```python
from build123d import *

# Parameters (mm, degrees)
F0_R      = 16.5
F1_DEPTH  = 10
F2_R      = 13
F3_DEPTH  = 10.5
F4_SIZE   = 0.5
F5_R      = 4.95
F6_DEPTH  = 12.5
F7_SIZE   = 0.5
F8_R      = 3.75
F9_DEPTH  = 8
F10_SIZE  = 0.5
F11_R     = 16.5
F11_R_2   = 13
F12_DEPTH = 7
F13_R     = 25
F14_DEPTH = 7
F15_SIZE  = 0.5


with BuildPart() as f1:
    # F0 (on Top) → F1 (new body)
    with BuildSketch(Plane.XY):
        Circle(F0_R)
    extrude(amount=F1_DEPTH)

    # F2 (on face) → F3 (join)
    with BuildSketch(Plane.XY.offset(10)):
        Circle(F2_R)
        with BuildLine():
            ThreePointArc((-7.4852813742, 6.6310302931), (-5, 8.6602540378), (-2, 9.7979589711))
            Line((-2, 9.7979589711), (-2, 8.4))
            Line((-2, 8.4), (2, 8.4))
            Line((2, 8.4), (2, 9.7979589711))
            ThreePointArc((2, 9.7979589711), (5, 8.6602540378), (7.4852813742, 6.6310302931))
            Line((7.4852813742, 6.6310302931), (6.2746133918, 5.9320508076))
            Line((6.2746133918, 5.9320508076), (8.2746133918, 2.4679491924))
            Line((8.2746133918, 2.4679491924), (9.4852813742, 3.166928678))
            ThreePointArc((9.4852813742, 3.166928678), (10, 0), (9.4852813742, -3.166928678))
            Line((9.4852813742, -3.166928678), (8.2746133918, -2.4679491924))
            Line((8.2746133918, -2.4679491924), (6.2746133918, -5.9320508076))
            Line((6.2746133918, -5.9320508076), (7.4852813742, -6.6310302931))
            ThreePointArc((7.4852813742, -6.6310302931), (5, -8.6602540378), (2, -9.7979589711))
            Line((2, -9.7979589711), (2, -8.4))
            Line((2, -8.4), (-2, -8.4))
            Line((-2, -8.4), (-2, -9.7979589711))
            ThreePointArc((-2, -9.7979589711), (-5, -8.6602540378), (-7.4852813742, -6.6310302931))
            Line((-7.4852813742, -6.6310302931), (-6.2746133918, -5.9320508076))
            Line((-6.2746133918, -5.9320508076), (-8.2746133918, -2.4679491924))
            Line((-8.2746133918, -2.4679491924), (-9.4852813742, -3.166928678))
            ThreePointArc((-9.4852813742, -3.166928678), (-10, 0), (-9.4852813742, 3.166928678))
            Line((-9.4852813742, 3.166928678), (-8.2746133918, 2.4679491924))
            Line((-8.2746133918, 2.4679491924), (-6.2746133918, 5.9320508076))
            Line((-6.2746133918, 5.9320508076), (-7.4852813742, 6.6310302931))
        make_face(mode=Mode.SUBTRACT)
    extrude(amount=F3_DEPTH)

    # F4
    f4_edges = [f1.edges().sort_by_distance(p)[0] for p in [
        (0, 8.4, 20.5),
        (-7.274613, 4.2, 20.5),
        (-7.274613, -4.2, 20.5),
        (0, -8.4, 20.5),
        (7.274613, -4.2, 20.5),
        (7.274613, 4.2, 20.5),
    ]]
    chamfer(f4_edges, length=F4_SIZE)

    # F5 (on face) → F6 (join)
    with BuildSketch(Plane.XY.offset(10)):
        Circle(F5_R)
    extrude(amount=F6_DEPTH)

    # F7
    f7_edges = [f1.edges().sort_by_distance(p)[0] for p in [
        (-4.95, 0, 22.5),
    ]]
    chamfer(f7_edges, length=F7_SIZE)

    # F8 (on face) → F9 (join)
    with BuildSketch(Plane.XY.offset(22.5)):
        Circle(F8_R)
    extrude(amount=F9_DEPTH)

    # F10
    f10_edges = [f1.edges().sort_by_distance(p)[0] for p in [
        (-3.75, 0, 30.5),
    ]]
    chamfer(f10_edges, length=F10_SIZE)

    # F11 (on face) → F12 (join)
    with BuildSketch(Plane.XY.offset(10)):
        Circle(F11_R)
        Circle(F11_R_2, mode=Mode.SUBTRACT)
    extrude(amount=F12_DEPTH)

    # F13 (on face) → F14 (cut)
    with BuildSketch(Plane(origin=(0, 0, 0), x_dir=(1, 0, 0), z_dir=(0, 0, -1))):
        Circle(F13_R)
    extrude(amount=-F14_DEPTH, mode=Mode.SUBTRACT)

    # F15
    f15_edges = [f1.edges().sort_by_distance(p)[0] for p in [
        (-13, 0, 20.5),
        (-16.5, 0, 17),
        (-16.5, 0, 7),
    ]]
    chamfer(f15_edges, length=F15_SIZE)


solid = f1.part
```
The listing builds one solid part. Answer for the finished solid, in the listing's coordinates (mm). A direction names the side the tool comes from. Give positions to 0.01 mm unless a question says otherwise; leave off trailing zeros. Loops run counter-clockwise (first coordinate to the right, second up) from the corner with the lowest first, then second, coordinate; pieces in that order, holes last. Notation, with made-up numbers: M 55.25,14.25 L 93.25,14.25 A20 ccw 93.25,48.25 Z; hole C -32.5,50 d2. An arc over 180 degrees is marked long. One line per item, written item: value.
Q1. For faces 1 (the face through (7.289, -4.176, 14.93)), 2 (the face through (0, 0, 7)), determine the directions among +Z, -Z, +X, -X, +Y, -Y from which every point of the face is accessible in a straight line to the end or side of a thin tool.
Working result:
face 1: +Z
face 2: -Z, +X, -X, +Y, -Y
Q2. A cutting plane is placed at B-B on z = 14. Determine the outline of the cut face in (x, y), then the cut area to 3 significant figures.
Working result:
outline: C 0,0 d33; C 0,0 d9.9; hole M -9.49,-3.17 L -8.27,-2.47 L -6.27,-5.93 L -7.49,-6.63 A10 ccw -2,-9.8 L -2,-8.4 L 2,-8.4 L 2,-9.8 A10 ccw 7.49,-6.63 L 6.27,-5.93 L 8.27,-2.47 L 9.49,-3.17 A10 ccw 9.49,3.17 L 8.27,2.47 L 6.27,5.93 L 7.49,6.63 A10 ccw 2,9.8 L 2,8.4 L -2,8.4 L -2,9.8 A10 ccw -7.49,6.63 L -6.27,5.93 L -8.27,2.47 L -9.49,3.17 A10 ccw Z
area: 655 mm^2
Q3. Determine the mould class of faces 3 (the face through (8.888, -2.822, 15.176)), 4 (the face through (0, 0, 30.5)), 5 (the face through (15.24, -6.32, 11.94)) for opening direction Y: +Y half, -Y half, draft (parallel to the pull), parting line (faces both ways), or undercut.
Working result:
face 3: undercut
face 4: draft
face 5: parting line
Q4. Find the intervals of material crossed by line 1 (Y direction, x = -7, z = 14.75); line 2 (Y direction, x = -6.5, z = 16.5); line 3 (Y direction, x = 3, z = 15), in increasing order. Write a range as from..to.
Working result:
line 1: y = -14.94..-7.14, -6.35..-4.68, 4.68..6.35, 7.14..14.94
line 2: y = -15.17..-7.6, -6.06..-5.54, 5.54..6.06, 7.6..15.17
line 3: y = -16.22..-9.54, -3.94..3.94, 9.54..16.22
Q5. Flat-ended cylindrical pins translate along their axes: P1, Ø2, axis at x = -9, y = 11.5, coming from the +Z side; P2, Ø3, axis at x = 0.5, z = 14, coming from the +Y side; P3, Ø5, axis at y = 11, z = 24.5, coming from the -X side; P4, Ø1, axis at x = 10, y = 5.5, coming from the +Z side. Find the tip coordinate at first contact, or state that the pin passes through.
Working result:
P1: stops at z = 17
P2: stops at y = 16.5
P3: passes through
P4: stops at z = 20.5
Q6. A cutting plane is placed at A-A on z = 19.25. Determine the outline of the cut face in (x, y), then the cut area to 3 significant figures.
Working result:
outline: C 0,0 d26; C 0,0 d9.9; hole M -9.49,-3.17 L -8.27,-2.47 L -6.27,-5.93 L -7.49,-6.63 A10 ccw -2,-9.8 L -2,-8.4 L 2,-8.4 L 2,-9.8 A10 ccw 7.49,-6.63 L 6.27,-5.93 L 8.27,-2.47 L 9.49,-3.17 A10 ccw 9.49,3.17 L 8.27,2.47 L 6.27,5.93 L 7.49,6.63 A10 ccw 2,9.8 L 2,8.4 L -2,8.4 L -2,9.8 A10 ccw -7.49,6.63 L -6.27,5.93 L -8.27,2.47 L -9.49,3.17 A10 ccw Z
area: 331 mm^2
